from build123d import *

# Parameters (mm, degrees)
F1_DEPTH = 0.2032
F2_DEPTH = 0.1016


with BuildPart() as f1:
    # F0 (on Front) → F1 (new body)
    with BuildSketch(Plane.XZ):
        Polygon((0, 18.0086), (9.801196, 18.0086), (11.01852, 39.9288), (0, 39.9288), (-11.01852, 39.9288), (-9.801196, 18.0086), align=None)
    extrude(amount=F1_DEPTH)

    # F0 (on Front) → F2 (join)
    with BuildSketch(Plane.XZ):
        Polygon((0, 39.9288), (11.01852, 39.9288), (12.4968, 66.548), (0, 66.548), (-12.4968, 66.548), (-11.01852, 39.9288), align=None)
        Polygon((-8.8011, 0), (0, 0), (8.8011, 0), (9.801196, 18.0086), (0, 18.0086), (-9.801196, 18.0086), align=None)
    extrude(amount=F2_DEPTH)


solid = f1.part
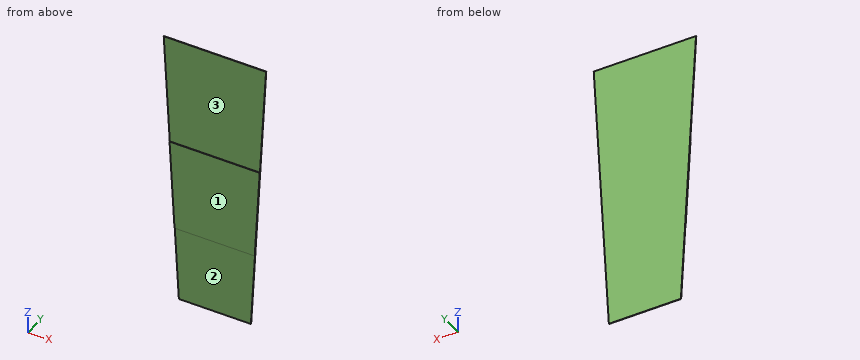
Geometry: final body of the model. Coordinates: model frame, mm. Face numbers are marked on the shaded views. A direction names the side the tool comes from. Give positions to 0.01 mm unless a question says otherwise; leave off trailing zeros. Write each loop counter-clockwise with the first axis right and the second up, starting at its lowest first coordinate (ties: lowest second). Pieces come first, ordered by that corner, then holes. Notation, with made-up numbers: M 85,17.5 L 121,17.5 A16 ccw 121,44.5 Z; hole C -39,47 d5. An arc over 180 degrees is marked long. Answer in a Markdown table with one row per item. Add a question column.
(1) Section C-C on z = 15.5. Return loops of the section in (x, y).
(2) Section B-B on x = 3.5. Return loops of the section in (y, z), and give its area (3 significant figures).
(3) Section A-A on y = -0.05. Return loops of the section in (x, z).
(4) First-contact query: pin 1 (1 mm diameter, centred on x = 4.5, z = 42.5, fed in from -Y); pin 2 (2 mm diameter, centred on x = -2, z = 30, fed in from +Y). Flat tips, straight axial feed; report the tip coordinate or a pass-through.
(5) Section D-D on z = 31. Return loops of the section in (x, y), and give its area (3 significant figures).
(6) Reachability of the marked faces 1, 2 and 3 from +Z, -Z, +X, -X, +Y, -Y: full face, straight path, thin tool, end or side. Return the list, or none.
(7) Ray query, line 1 (Z direction, x = 3.75, y = -0.15); line 2 (X direction, y = -0.05, z = 63.5); line 3 (X direction, y = -0.05, z = 7.5). Return the intervals inside material, ascending.
Result set:
| question | item | result |
|---|---|---|
| 1 | outline | M -9.66,-0.1 L 9.66,-0.1 L 9.66,0 L -9.66,0 Z |
| 2 | outline | M -0.2,18.01 L -0.1,18.01 L -0.1,0 L 0,0 L 0,66.55 L -0.1,66.55 L -0.1,39.93 L -0.2,39.93 Z |
| 2 | area | 8.99 mm^2 |
| 3 | outline | M -12.5,66.55 L -8.8,0 L 8.8,0 L 12.5,66.55 Z |
| 4 | pin 1 | stops at y = -0.1 |
| 4 | pin 2 | stops at y = 0 |
| 5 | outline | M -10.52,-0.2 L 10.52,-0.2 L 10.52,0 L -10.52,0 Z |
| 5 | area | 4.28 mm^2 |
| 6 | face 1 | +Z, -Z, +X, -X, -Y |
| 6 | face 2 | -Z, +X, -X, -Y |
| 6 | face 3 | +Z, +X, -X, -Y |
| 7 | line 1 | z = 18.01 to 39.93 |
| 7 | line 2 | x = -12.33 to 12.33 |
| 7 | line 3 | x = -9.22 to 9.22 |
